Part model, mm, in its own coordinate system. Face numbers are marked on the shaded views. Round coordinates to 2 decimals unless told otherwise and drop trailing zeros. Write each loop counter-clockwise with the first axis right and the second up, starting at its lowest first coordinate (ties: lowest second). Pieces come first, ordered by that corner, then holes. Notation, with made-up numbers: (89, 21) -> (119, 21) arc R23 cw to (119, 60) -> close; hole circle Ø8 at (20, 12.5). An arc over 180 degrees is marked (long way). Use CSV: the item, a comma, the result in double quotes. Start each with the question number.
(1) Saw through at D-D (z = 4). Give the cut face in (x, y), plus the area to 3 significant figures.
(2) Saw through at C-C (x = -5.2). Give the cut face in (y, z).
(3) Two-plate mould, pull along X, no slides. Class the marked faces 1, 2, 3 and 4: released by +X, released by -X, zero draft, split by the parting line, or undercut.
(4) Saw through at B-B (y = 0). Give the cut face in (x, z), plus the area to 3 significant figures.
(5) Drop flat-ended pins along their axis: pin 1 (5 mm diameter, centred on x = -5.2, y = 37.02, fed in from -Z); pin 2 (3 mm diameter, centred on y = 17, z = 2, fed in from -X). Give the stop position or say it passes through.
(6) Saw through at A-A (x = -0.5). Give the cut face in (y, z), plus the area to 3 significant figures.
(7) Probe line 1 (Y direction, x = 0, z = 4.7); line 2 (Y direction, x = 1, z = 5.5); line 3 (Y direction, x = -5.2, z = 2.7). List the from-to ranges inside material, lowest first. Write a range as [from, to].
```python
from build123d import *

# Parameters (mm, degrees)
SKETCH1_R               = 7.95
SKETCH1_R_2             = 3
MAIN_BODY_LINK_B2_DEPTH = 6
CUT_EXTRUDE1_REACH      = 48.699
SKETCH2_R               = 1.5
CUT_EXTRUDE2_DEPTH      = 47.698679231
SKETCH4_R               = 15.25
CUT_EXTRUDE3_DEPTH      = 47.698679231


with BuildPart() as part:
    # Sketch1 → Main Body Link B2 (new body)
    with BuildSketch(Plane.XY):
        with BuildLine():
            Line((0, 41.674052381), (20.2, 41.674052381))
            Line((20.2, 41.674052381), (20.2, 34.274052381))
            Line((20.2, 34.274052381), (17.964224051, -1.134307826))
            ThreePointArc((17.964224051, -1.134307826), (0, -18), (-17.964224051, -1.134307826))
            Line((-17.964224051, -1.134307826), (-20.2, 34.274052381))
            Line((-20.2, 34.274052381), (-20.2, 41.674052381))
            Line((-20.2, 41.674052381), (0, 41.674052381))
        make_face()
        Circle(SKETCH1_R, mode=Mode.SUBTRACT)
        with Locations((-15, 37.024052381)):
            Circle(SKETCH1_R_2, mode=Mode.SUBTRACT)
        with Locations((-5.2, 37.024052381)):
            Circle(SKETCH1_R_2, mode=Mode.SUBTRACT)
        with Locations((5.2, 37.024052381)):
            Circle(SKETCH1_R_2, mode=Mode.SUBTRACT)
        with Locations((15, 37.024052381)):
            Circle(SKETCH1_R_2, mode=Mode.SUBTRACT)
    extrude(amount=MAIN_BODY_LINK_B2_DEPTH)

    # Sketch2 → Cut-Extrude1 (cut, up to next)
    with BuildSketch(Plane.XY.offset(6), mode=Mode.PRIVATE) as cut_extrude1_sk1:
        with Locations((-11.5, 0)):
            Circle(SKETCH2_R)
    cut_extrude1_tool1 = extrude(cut_extrude1_sk1.sketch, amount=-CUT_EXTRUDE1_REACH, mode=Mode.PRIVATE) & part.part
    # Sketch2 → Cut-Extrude1 (cut, up to next)
    with BuildSketch(Plane.XY.offset(6), mode=Mode.PRIVATE) as cut_extrude1_sk2:
        with Locations((11.5, 0)):
            Circle(SKETCH2_R)
    cut_extrude1_tool2 = extrude(cut_extrude1_sk2.sketch, amount=-CUT_EXTRUDE1_REACH, mode=Mode.PRIVATE) & part.part
    add(cut_extrude1_tool1.solids().sort_by_distance((-11.5, 0, 6))[0], mode=Mode.SUBTRACT)
    add(cut_extrude1_tool2.solids().sort_by_distance((11.5, 0, 6))[0], mode=Mode.SUBTRACT)

    # Sketch3 → Cut-Extrude2 (cut, through all)
    with BuildSketch(Plane.XY.offset(6)):
        with BuildLine():
            Line((-8.682671659, 28.521221325), (3.604609006, 19.91757478))
            ThreePointArc((3.604609006, 19.91757478), (4.095760221, 17.132117818), (1.31030326, 16.640966602))
            Line((1.31030326, 16.640966602), (-10.976977404, 25.244613148))
            ThreePointArc((-10.976977404, 25.244613148), (-11.46812862, 28.030070109), (-8.682671659, 28.521221325))
        make_face()
    extrude(amount=-CUT_EXTRUDE2_DEPTH, mode=Mode.SUBTRACT)

    # Sketch4 → Cut-Extrude3 (cut, through all)
    with BuildSketch(Plane.XY.offset(6)):
        Circle(SKETCH4_R)
    extrude(amount=-CUT_EXTRUDE3_DEPTH, mode=Mode.SUBTRACT)


solid = part.part
```
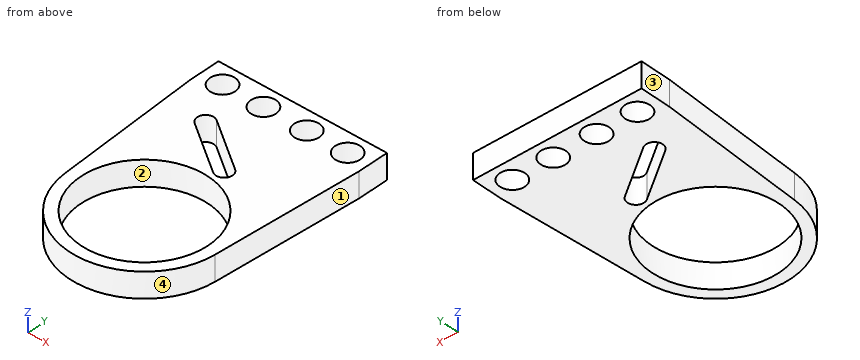
Answers:
1,outline,"(-20.2, 34.27) -> (-17.96, -1.13) arc R18 ccw to (17.96, -1.13) -> (20.2, 34.27) -> (20.2, 41.67) -> (-20.2, 41.67) -> close; hole circle Ø6 at (-15, 37.02); hole circle Ø30.5 at (0, 0); hole (-10.98, 25.24) -> (1.31, 16.64) arc R2 ccw to (3.6, 19.92) -> (-8.68, 28.52) arc R2 ccw to start; hole circle Ø6 at (-5.2, 37.02); hole circle Ø6 at (5.2, 37.02); hole circle Ø6 at (15, 37.02)"
1,area,"1,200 mm²"
2,outline,"(-17.23, 0) -> (-14.34, 0) -> (-14.34, 6) -> (-17.23, 6) -> close; (14.34, 0) -> (21.2, 0) -> (21.2, 6) -> (14.34, 6) -> close; (26.08, 0) -> (34.02, 0) -> (34.02, 6) -> (26.08, 6) -> close; (40.02, 0) -> (41.67, 0) -> (41.67, 6) -> (40.02, 6) -> close"
3,face 1,"released by +X"
3,face 2,"undercut"
3,face 3,"released by -X"
3,face 4,"split by the parting line"
4,outline,"(-18.04, 0) -> (-15.25, 0) -> (-15.25, 6) -> (-18.04, 6) -> close; (15.25, 0) -> (18.04, 0) -> (18.04, 6) -> (15.25, 6) -> close"
4,area,"33.4 mm²"
5,pin 1,"passes through"
5,pin 2,"stops at x = -19.2"
6,outline,"(-17.99, 0) -> (-15.24, 0) -> (-15.24, 6) -> (-17.99, 6) -> close; (15.24, 0) -> (17.91, 0) -> (17.91, 6) -> (15.24, 6) -> close; (22.79, 0) -> (41.67, 0) -> (41.67, 6) -> (22.79, 6) -> close"
6,area,"146 mm²"
7,line 1,"y = [-18, -15.25], [15.25, 17.56], [22.44, 41.67]"
7,line 2,"y = [-17.97, -15.22], [15.22, 16.86], [21.74, 41.67]"
7,line 3,"y = [-17.23, -14.34], [14.34, 21.2], [26.08, 34.02], [40.02, 41.67]"
